```python
from build123d import *

# Parameters (mm, degrees)
SKETCH_1_R               = 18.5
EXTRUDE_1_DEPTH          = 23
SKETCH_2_R               = 16.5
EXTRUDE_2_DEPTH          = 23
SKETCH_3_R               = 6
EXTRUDE_3_DEPTH          = 6
SKETCH_4_R               = 3
EXTRUDE_4_DEPTH          = 12
CUT_EXTRUDE_1_DEPTH      = 53.919750566
CUT_EXTRUDE_1_DEPTH_BACK = 53.919750566
SKETCH_5_W               = 8.515862451
SKETCH_5_H               = 10.43869594
SKETCH_6_R               = 1
EXTRUDE_5_DEPTH          = 2
SKETCH_7_R               = 16.5
EXTRUDE_6_DEPTH          = 2
SKETCH_8_R               = 7.139531777
EXTRUDE_7_DEPTH          = 5
SKETCH_9_W               = 20.48733328
SKETCH_9_H               = 9.95175006
EXTRUDE_8_DEPTH          = 6
SKETCH_10_R              = 1.5
CUT_EXTRUDE_2_DEPTH      = 2


with BuildPart() as part:
    # 草图1 → 凸台-拉伸1 (new body)
    with BuildSketch(Plane.XY):
        Circle(SKETCH_1_R)
    extrude(amount=EXTRUDE_1_DEPTH)

    # 草图2 → 凸台-拉伸2 (add)
    with BuildSketch(Plane.XY.offset(23)):
        Circle(SKETCH_2_R)
    extrude(amount=EXTRUDE_2_DEPTH)

    # 草图3 → 凸台-拉伸3 (add)
    with BuildSketch(Plane(origin=(0, 0, 0), x_dir=(-1, 0, 0), z_dir=(0, 0, -1))):
        with Locations(Location((0, 7, 0), (0, 0, 180))):
            Circle(SKETCH_3_R)
    extrude(amount=EXTRUDE_3_DEPTH)

    # 草图4 → 凸台-拉伸4 (add)
    with BuildSketch(Plane(origin=(0, 0, -6), x_dir=(-1, 0, 0), z_dir=(0, 0, -1))):
        with Locations((0, 7)):
            Circle(SKETCH_4_R)
    extrude(amount=EXTRUDE_4_DEPTH)

    # 草图5 → 切除-拉伸1 (cut, two sides: drawn at the far end of the back side and taken through both)
    with BuildSketch(Plane(origin=(0, 0, 0), x_dir=(0, 0, -1), z_dir=(1, 0, 0)).offset(-CUT_EXTRUDE_1_DEPTH_BACK)):
        with Locations((15.772473003, 14.71934797)):
            Rectangle(SKETCH_5_W, SKETCH_5_H)
    extrude(amount=CUT_EXTRUDE_1_DEPTH + CUT_EXTRUDE_1_DEPTH_BACK, mode=Mode.SUBTRACT)

    # 草图6 → 凸台-拉伸5 (add)
    with BuildSketch(Plane.XY.offset(46)):
        with Locations((-10, 0)):
            Circle(SKETCH_6_R)
        with Locations((10, 0)):
            Circle(SKETCH_6_R)
    extrude(amount=EXTRUDE_5_DEPTH)

    # 草图7 → 凸台-拉伸6 (add)
    with BuildSketch(Plane.XY.offset(48)):
        Circle(SKETCH_7_R)
    extrude(amount=EXTRUDE_6_DEPTH)

    # 草图8 → 凸台-拉伸7 (add)
    with BuildSketch(Plane.XY.offset(50)):
        Circle(SKETCH_8_R)
    extrude(amount=EXTRUDE_7_DEPTH)

    # 草图9 → 凸台-拉伸8 (add)
    with BuildSketch(Plane.XY.offset(50)):
        with Locations((0, 16.5)):
            Rectangle(SKETCH_9_W, SKETCH_9_H)
    extrude(amount=EXTRUDE_8_DEPTH)

    # 草图10 → 切除-拉伸2 (cut)
    with BuildSketch(Plane(origin=(0, 0, 0), x_dir=(-1, 0, 0), z_dir=(0, 0, -1))):
        with Locations((15.5, 0)):
            Circle(SKETCH_10_R)
        with Locations((7.75, -13.423393759)):
            Circle(SKETCH_10_R)
        with Locations((-7.75, -13.423393759)):
            Circle(SKETCH_10_R)
        with Locations((-15.5, 0)):
            Circle(SKETCH_10_R)
        with Locations((-7.75, 13.423393759)):
            Circle(SKETCH_10_R)
        with Locations((7.75, 13.423393759)):
            Circle(SKETCH_10_R)
    extrude(amount=-CUT_EXTRUDE_2_DEPTH, mode=Mode.SUBTRACT)


solid = part.part
```
Can you work these out from the model? Positions are in its coordinate system, mm. A direction names the side the tool comes from. Round coordinates to 2 decimals unless told otherwise and drop trailing zeros. Loops run counter-clockwise (first coordinate to the right, second up) from the corner with the lowest first, then second, coordinate; pieces in that order, holes last. Notation, with made-up numbers: M -29,42 L -15,42 A24 ccw -15,77 Z; hole C -1,83 d10. An arc over 180 degrees is marked long. Write item = value, one per line. Start each with the question number.
(1) Suppose I cut it at D-D on z = 36. Write out the boundary of the cut face in (x, y).
(2) I'm going to push flat-ended pins straight in: P1, Ø4, axis at x = -15.5, y = 0, coming from the +Z side; P2, Ø4.5, axis at x = -3.5, y = 18.5, coming from the -Z side; P3, Ø1.8, axis at y = 19, z = 53.5, coming from the -X side. Where does each tip first touch, or does it pass through?
(3) If we mould it in two halves opening along Y, with no side actions, what happens to faces 1 (the face through (-17, 0, 23)), 2 (the face through (8, 13, 2)), 3 (the face through (0, 21.476, 53))? For each: released by +Y, released by -Y, zero draft, split by the parting line, or undercut.
(4) Suppose I cut it at C-C on y = 5. Write out the boundary of the cut face in (x, z).
(5) Which directions (+Z, -Z, +X, -X, +Y, -Y) give clear straight access to the entire face, cutting with the end or side of a thin tool? Please do faces 4 (the face through (0, 11.524, 53)), 5 (the face through (15.24, -6.32, 48.99)), 6 (the face through (17, 0, 1)), 7 (the face through (10.244, 16, 53)), 8 (the face through (-10.244, 16, 53)).
(6) I need wall thicknesses on line 1 along Z through (x, y) = (-2.5, 12); line 2 along Z through (x, y) = (1, -4); line 3 along Y through (x, z) = (-7.75, 1.35). Which ranges of each line are inside material? Lowest first, please.
Answer block:
q1.outline = C 0,0 d33
q2.P1 = 50
q2.P2 = 0
q2.P3 = -10.24
q3.face_1 = zero draft
q3.face_2 = undercut
q3.face_3 = released by +Y
q4.outline = M -17.81,0 L -5.66,0 L -5.66,-6 L -2.24,-6 L -2.24,-18 L 2.24,-18 L 2.24,-6 L 5.66,-6 L 5.66,0 L 17.81,0 L 17.81,23 L 15.72,23 L 15.72,46 L -15.72,46 L -15.72,23 L -17.81,23 Z; M -15.72,48 L 15.72,48 L 15.72,50 L 5.1,50 L 5.1,55 L -5.1,55 L -5.1,50 L -15.72,50 Z
q5.face_4 = +Z, +X, -X
q5.face_5 = none
q5.face_6 = -Z
q5.face_7 = +Z, +X, +Y, -Y
q5.face_8 = +Z, -X, +Y, -Y
q6.line_1 = -6 to 46, 48 to 56
q6.line_2 = 0 to 46, 48 to 55
q6.line_3 = -16.8 to -14.92, -11.92 to 11.92, 14.92 to 16.8
